from build123d import *

# Parameters (mm, degrees)
SKETCH1_R           = 6
SKETCH1_R_2         = 4
BOSS_EXTRUDE1_DEPTH = 12.5
SKETCH2_R           = 6
SKETCH2_R_2         = 4
BOSS_EXTRUDE2_DEPTH = 15
CUT_EXTRUDE1_START  = -25
SKETCH3_R           = 4
CUT_EXTRUDE1_DEPTH  = 25


with BuildPart() as part:
    # Sketch1 → Boss-Extrude1 (new, symmetric)
    with BuildSketch(Plane.XY):
        Circle(SKETCH1_R)
        Circle(SKETCH1_R_2, mode=Mode.SUBTRACT)
    extrude(amount=BOSS_EXTRUDE1_DEPTH, both=True)

    # Sketch2 → Boss-Extrude2 (add)
    with BuildSketch(Plane(origin=(0, 0, 0), x_dir=(1, 0, 0), z_dir=(0, 1, 0))):
        Circle(SKETCH2_R)
        with Locations(Location((0, 0, 0), (0, 0, 90))):
            Circle(SKETCH2_R_2, mode=Mode.SUBTRACT)
    extrude(amount=BOSS_EXTRUDE2_DEPTH)

    # Sketch3 → Cut-Extrude1 (cut)
    with BuildSketch(Plane.XY.offset(12.5).offset(CUT_EXTRUDE1_START)):
        Circle(SKETCH3_R)
    extrude(amount=CUT_EXTRUDE1_DEPTH, mode=Mode.SUBTRACT)


solid = part.part
Work out the finished part from the listing and answer in its coordinate system (mm). A direction names the side the tool comes from. Round coordinates to 2 decimals unless told otherwise and drop trailing zeros. Write each loop counter-clockwise with the first axis right and the second up, starting at its lowest first coordinate (ties: lowest second). Pieces come first, ordered by that corner, then holes.
1) A cutting plane is placed at D-D (y = 11.5). Give the vertices of the cut face in (x, z), plus the area to 3 significant figures.
2) A cutting plane is placed at A-A (x = 0). Give the vertices of the cut face in (y, z), plus the area to 3 significant figures.
3) A tool of negligible diameter and unlimited length cuts with its end or side. For faces 1 (the flat face through (-1.42, -3.92, 12.5)), 2 (the cylindrical face through (-1.301, -5.857, 0.175)), from which of +Z, -Z, +X, -X, +Y, -Y can it reach the whole face along a straight path? Write none if from no direction.
4) Straight lines are drawn through the part: line 1 (Y direction, x = 0, z = -0.25); line 2 (X direction, y = -2, z = -7.75). For each, find the intervals that lie inside material, in ascending order.
5) The mould has two halves that part along X. Classify faces 3 (the flat face through (-1.42, -3.92, -12.5)), 4 (the cylindrical face through (1.532, 9.662, -3.695)), 5 (the cylindrical face through (-6, 9, 0)): pulls with the +X half, pulls with the -X half, needs draft (parallel to the pull), parting line crosses it, or undercut.
6) Given pin 1 Ø1.5 at (x, z) = (4.5, -9.5) entering from +Y; pin 2 Ø1 at (x, z) = (-0.5, 5) entering from -Y; pin 3 Ø3 at (y, z) = (3.5, -4.5) entering from -X, each flat-ended and moving along its own axis, determine where each tip first touches the part or whether it passes through.
7) A cutting plane is placed at B-B (z = 0). Give the vertices of the cut face in (x, y).
8) A cutting plane is placed at C-C (y = 1). Give the vertices of the cut face in (x, z), plus the area to 3 significant figures.
Completed:
1. outline: circle Ø12 at (0, 0); hole circle Ø8 at (0, 0)
1. area: 62.8 mm2
2. outline: (-6, -12.5) - (-4, -12.5) - (-4, 12.5) - (-6, 12.5) - close; (4, -12.5) - (6, -12.5) - (6, -6) - (15, -6) - (15, -4) - (6, -4) - (6, 4) - (15, 4) - (15, 6) - (6, 6) - (6, 12.5) - (4, 12.5) - close
2. area: 136 mm2
3. face 1: +Z, +X, -X, +Y, -Y
3. face 2: none
4. line 1: y = -6 to -4, 4 to 6
4. line 2: x = -5.66 to -3.46, 3.46 to 5.66
5. face 3: needs draft
5. face 4: undercut
5. face 5: parting line crosses it
6. pin 1: stops at y = 4.68
6. pin 2: stops at y = -6
6. pin 3: stops at x = -5.66
7. outline: (-6, 0) arc R6 ccw to (6, 0) - (6, 15) - (4, 15) - (4, 4.47) arc R6 ccw to (-4, 4.47) - (-4, 15) - (-6, 15) - close; hole circle Ø8 at (0, 0)
8. outline: (-5.92, -12.5) - (-3.87, -12.5) - (-3.87, 12.5) - (-5.92, 12.5) - (-5.92, 1) arc R6 ccw to (-5.92, -1) - close; (3.87, -12.5) - (5.92, -12.5) - (5.92, -1) arc R6 ccw to (5.92, 1) - (5.92, 12.5) - (3.87, 12.5) - close
8. area: 102 mm2
